from build123d import *

# Parameters (mm, degrees)
SKETCH1_R           = 1.5
BOSS_EXTRUDE1_DEPTH = 5
SKETCH2_W           = 8
SKETCH2_H           = 5
CUT_EXTRUDE1_DEPTH  = 10
SKETCH3_R           = 1.5
CUT_EXTRUDE2_DEPTH  = 10
CUT_EXTRUDE4_DEPTH  = 10


with BuildPart() as part:
    # Sketch1 → Boss-Extrude1 (new body)
    with BuildSketch(Plane.XY):
        with BuildLine():
            Line((-12.5, 0), (-12.5, -77.5))
            Line((-12.5, -77.5), (12.5, -77.5))
            Line((12.5, -77.5), (12.5, 0))
            ThreePointArc((12.5, 0), (0, 12.5), (-12.5, 0))
        make_face()
        Circle(SKETCH1_R, mode=Mode.SUBTRACT)
        with Locations((0, 7)):
            Circle(SKETCH1_R, mode=Mode.SUBTRACT)
        with Locations((4.949747468, 4.949747468)):
            Circle(SKETCH1_R, mode=Mode.SUBTRACT)
        with Locations((7, 0)):
            Circle(SKETCH1_R, mode=Mode.SUBTRACT)
        with Locations((4.949747468, -4.949747468)):
            Circle(SKETCH1_R, mode=Mode.SUBTRACT)
        with Locations((0, -7)):
            Circle(SKETCH1_R, mode=Mode.SUBTRACT)
        with Locations((-4.949747468, -4.949747468)):
            Circle(SKETCH1_R, mode=Mode.SUBTRACT)
        with Locations((-7, 0)):
            Circle(SKETCH1_R, mode=Mode.SUBTRACT)
        with Locations((-4.949747468, 4.949747468)):
            Circle(SKETCH1_R, mode=Mode.SUBTRACT)
    extrude(amount=BOSS_EXTRUDE1_DEPTH)

    # Sketch2 → Cut-Extrude1 (cut)
    with BuildSketch(Plane.XY.offset(5)):
        with Locations((0, -43)):
            Rectangle(SKETCH2_W, SKETCH2_H)
    extrude(amount=-CUT_EXTRUDE1_DEPTH, mode=Mode.SUBTRACT)

    # Sketch3 → Cut-Extrude2 (cut)
    with BuildSketch(Plane.XY.offset(5)):
        with Locations((0, -65)):
            Circle(SKETCH3_R)
        with Locations((0, -58)):
            Circle(SKETCH3_R)
        with Locations((-7, -65)):
            Circle(SKETCH3_R)
        with Locations((7, -65)):
            Circle(SKETCH3_R)
        with Locations((0, -72)):
            Circle(SKETCH3_R)
    extrude(amount=-CUT_EXTRUDE2_DEPTH, mode=Mode.SUBTRACT)

    # Sketch4 → Cut-Extrude4 (cut)
    with BuildSketch(Plane.XY.offset(5)):
        with BuildLine():
            Line((5, -20), (5, -28))
            Line((5, -28), (12.5, -35.5))
            Line((12.5, -35.5), (12.5, -27.5))
            ThreePointArc((12.5, -27.5), (17.803300859, -14.696699141), (5, -20))
        make_face()
    extrude(amount=-CUT_EXTRUDE4_DEPTH, mode=Mode.SUBTRACT)


solid = part.part
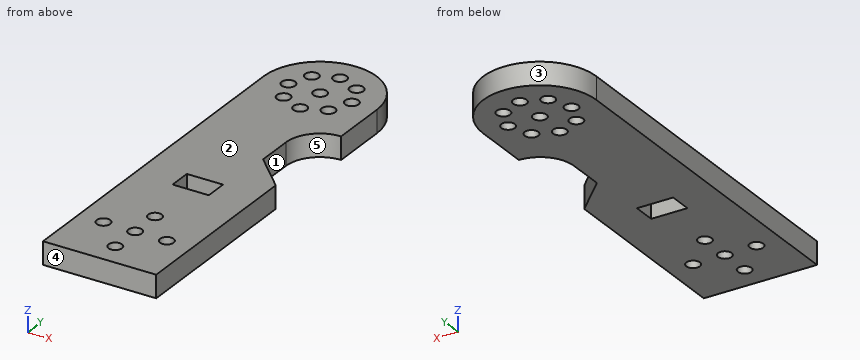
Can you work these out from the model? Positions are in its coordinate system, mm. Face numbers are marked on the shaded views. A direction names the side the tool comes from. Coordinates: 2 decimals unless noted, no trailing zeros. Loops run counter-clockwise (first coordinate to the right, second up) from the corner with the lowest first, then second, coordinate; pieces in that order, holes last. Notation, with made-up numbers: M 72.5,16 L 100.5,16 A23 ccw 100.5,47 Z; hole C -5.75,22 d11. An arc over 180 degrees is marked long. Return JSON: item names as keys, results as strings. Group by question number.
Item 1: If I drill on L1, parallel to X at y = -65, z = 1.8; L2, parallel to X at y = -45, z = 2.05; L3, parallel to X at y = -5, z = 3.2, over which ranges is the centre line in solid material (lowest first)? Write a range as from..to.
Item 2: Imagine slicing it at A-A (y = -58). Please give me the cut outline in (x, z).
Item 3: Imagine slicing it at D-D (x = 7.75). Please give me the cut outline in (y, z).
Item 4: Imagine slicing it at B-B (x = 0). Give the number of separate pieces and of enclosed holes in the cut face, and give its area (3 significant figures).
Item 5: Thinking about a two-plate mould opening in Y: for the marked faces 1, 2 and 3, which applies, released by +Y, released by -Y, zero draft, split by the parting line, or undercut?
Item 6: On a 3-axis mill with a long thin cutter (end or side, diameter ignored), from which of +Z, -Z, +X, -X, +Y, -Y can I reach the whole of each face in a straight line? I mean the marked faces 4 and 5. Say none if no direction works.
Verdict:
{
 "1": {"L1": "x = -12.5..-8.5, -5.5..-1.5, 1.5..5.5, 8.5..12.5", "L2": "x = -12.5..-4, 4..12.5", "L3": "x = -12.5..-6.45, -3.45..3.45, 6.45..12.5"},
 "2": {"outline": "M -12.5,0 L -1.5,0 L -1.5,5 L -12.5,5 Z; M 1.5,0 L 12.5,0 L 12.5,5 L 1.5,5 Z"},
 "3": {"outline": "M -77.5,0 L -66.3,0 L -66.3,5 L -77.5,5 Z; M -63.7,0 L -30.75,0 L -30.75,5 L -63.7,5 Z; M -14.2,0 L -1.3,0 L -1.3,5 L -14.2,5 Z; M 1.3,0 L 9.81,0 L 9.81,5 L 1.3,5 Z"},
 "4": {"separate pieces": "8", "enclosed holes": "0", "area": "335 mm^2"},
 "5": {"face 1": "undercut", "face 2": "zero draft", "face 3": "released by +Y"},
 "6": {"face 4": "+Z, -Z, +X, -X, -Y", "face 5": "+Z, -Z, +X"}
}
